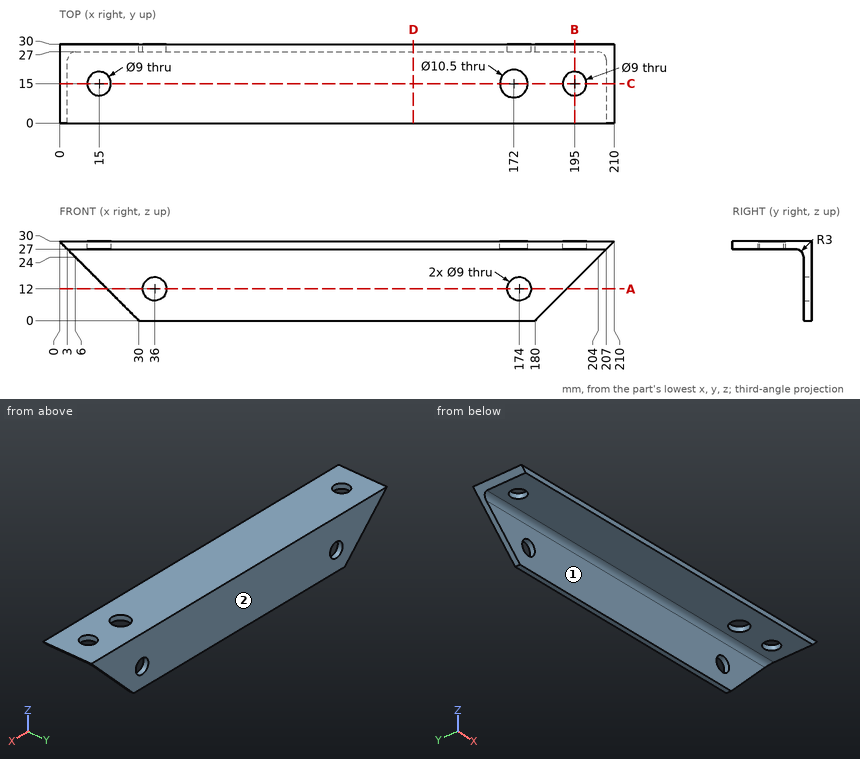
Verification items for this drawing (mm, ordinates from the low corner). A direction names the side the tool comes from. Give positions to 0.01 mm unless a question says otherwise; leave off trailing zeros. Loops run counter-clockwise (first coordinate to the right, second up) from the corner with the lowest first, then second, coordinate; pieces in that order, holes last. Notation, with made-up numbers: M 30.5,16 L 58.5,16 A13 cw 58.5,30 Z; hole C 78.25,-39.75 d7. An arc over 180 degrees is marked long. Answer as a JSON object with one key per item and string values. Group by question number.
Q1. Material ranges on line 1 along Y through (x, z) = (172, 28.5); line 2 along Y through (x, z) = (195, 29); line 3 along Z through (x, y) = (36, 27.95), recorded low to high. Write a range as [from, to].
Q2. Cross-section at A-A on z = 12. Record the cut outline in (x, y), then the cut area to 3 significant figures.
Q3. Go/stop test with flat-tipped pins: P1, Ø5, axis at x = 54, z = 18, coming from the -Y side; P2, Ø1, axis at x = 155.5, y = 14.5, coming from the -Z side; P3, Ø14.5, axis at x = 195, y = 15, coming from the +Z side; P4, Ø7, axis at x = 36, z = 12, coming from the -Y side. Record where each tip stops, or that it passes through.
Q4. Cross-section at C-C on y = 15. Record the cut outline in (x, z), then the cut area to 4 significant figures.
Q5. Access from +Z, -Z, +X, -X, +Y, -Y to the whole of each face (thin tool, end or side, straight path). Record for the marked faces 1 and 2.
Q6. Cross-section at B-B on x = 195. Record the cut outline in (y, z).
Q7. Cross-section at D-D on x = 134. Record the cut outline in (y, z).
Evaluation:
{
 "1": {"line 1": "y = [0, 9.75], [20.25, 30]", "line 2": "y = [0, 10.5], [19.5, 30]", "line 3": "z = [0, 7.5], [16.5, 30]"},
 "2": {"outline": "M 18,27 L 31.5,27 L 31.5,30 L 18,30 Z; M 40.5,27 L 169.5,27 L 169.5,30 L 40.5,30 Z; M 178.5,27 L 192,27 L 192,30 L 178.5,30 Z", "area": "468 mm2"},
 "3": {"P1": "stops at y = 27", "P2": "stops at z = 27", "P3": "stops at z = 30", "P4": "passes through"},
 "4": {"outline": "M 0,30 L 3,27 L 10.5,27 L 10.5,30 Z; M 19.5,27 L 166.75,27 L 166.75,30 L 19.5,30 Z; M 177.25,27 L 190.5,27 L 190.5,30 L 177.25,30 Z; M 199.5,27 L 207,27 L 210,30 L 199.5,30 Z", "area": "535.5 mm2"},
 "5": {"face 1": "-Z, +X, -X, -Y", "face 2": "+Z, -Z, +X, -X, +Y"},
 "6": {"outline": "M 0,27 L 10.5,27 L 10.5,30 L 0,30 Z; M 19.5,27 L 24,27 A3 cw 27,24 L 27,15 L 30,15 L 30,30 L 19.5,30 Z"},
 "7": {"outline": "M 0,27 L 24,27 A3 cw 27,24 L 27,0 L 30,0 L 30,30 L 0,30 Z"}
}
